```python
from build123d import *

# Parameters (mm, degrees)
SKETCH_1_W      = 15
SKETCH_1_H      = 3
EXTRUDE_1_DEPTH = 3
CHAMFER_1_SIZE  = 1


with BuildPart() as part:
    # Эскиз1 → Бобышка-Вытянуть1 (new body)
    with BuildSketch(Plane(origin=(0, 0, 0), x_dir=(1, 0, 0), z_dir=(0, 1, 0))):
        Rectangle(SKETCH_1_W, SKETCH_1_H)
    extrude(amount=EXTRUDE_1_DEPTH)

    # Фаска1
    chamfer_1_edges = [part.edges().sort_by_distance(p)[0] for p in [
        (0, 3, -1.5),
    ]]
    chamfer(chamfer_1_edges, length=CHAMFER_1_SIZE)


solid = part.part
```
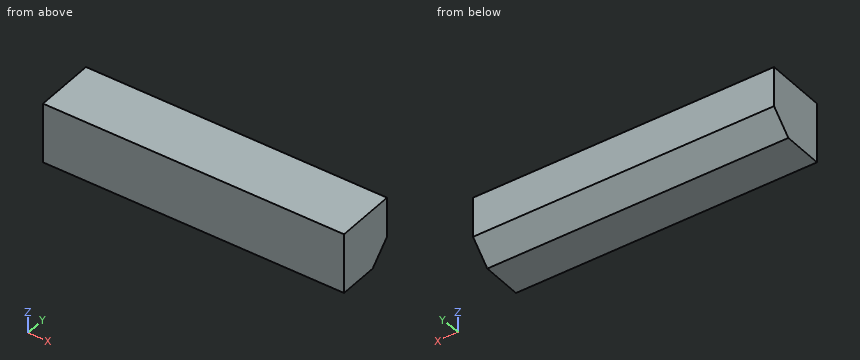
Model file for the job. Use its own axes, mm. Round coordinates to 2 decimals unless told otherwise and drop trailing zeros. Order: outer loops, then holes, each group sorted by start corner. A loop starts at its lowest first (then second) coordinate and runs counter-clockwise, first axis right, second up. Notation, with made-up numbers: M 0.5,-22.5 L 36.5,-22.5 A27 ccw 36.5,14.5 Z; hole C 42,41.5 d5. An arc over 180 degrees is marked long. Use CSV: the item, a comma, the result in double quotes.
Item 1: Saw through at A-A (x = 5). List the corners of the cut face in (y, z).
Worked answers:
outline,"M 0,-1.5 L 2,-1.5 L 3,-0.5 L 3,1.5 L 0,1.5 Z"
Item 2: Saw through at C-C (y = 2.8). List the corners of the cut face in (x, z).
Worked answers:
outline,"M -7.5,-0.7 L 7.5,-0.7 L 7.5,1.5 L -7.5,1.5 Z"
Item 3: Probe probe 1 along Z at (x, y) = (5.5, 2.6); probe 2 along Y at (x, z) = (-4.5, -0.55); probe 3 along Y at (x, z) = (-4.25, -1.05). List the from-to ranges inside material, lowest first.
Worked answers:
probe 1,"-0.9 to 1.5"
probe 2,"0 to 2.95"
probe 3,"0 to 2.45"
Item 4: Saw through at B-B (z = -0.9). List the corners of the cut face in (x, y), plus the area to 3 significant figures.
Worked answers:
outline,"M -7.5,0 L 7.5,0 L 7.5,2.6 L -7.5,2.6 Z"
area,"39.0 mm²"
